Source: CAD feature listing. Evaluate the final solid. Frame: model axes, mm. Face numbers are marked on the shaded views. Round coordinates to 2 decimals unless told otherwise and drop trailing zeros. Write each loop counter-clockwise with the first axis right and the second up, starting at its lowest first coordinate (ties: lowest second). Pieces come first, ordered by that corner, then holes. Notation, with made-up numbers: M 85,-18.75 L 139,-18.75 A14 ccw 139,7.25 Z; hole C 73.25,41.5 d8. An arc over 180 degrees is marked long. Use a Markdown table: item, result.
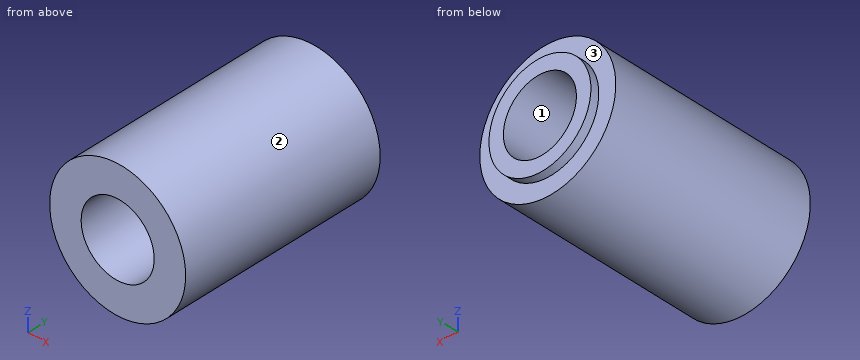
```python
from build123d import *

# Parameters (mm, degrees)
SKETCH1_R            = 4
BOSS_EXTRUDE1_DEPTH  = 12.82
SKETCH2_OUTSIDE_W    = 13.42
SKETCH2_OUTSIDE_H    = 13.42
SKETCH2_OUTSIDE_R    = 3
CUT_EXTRUDE1_DEPTH   = 0.5
M4_CLEARANCE_HOLE1_D = 4.3


with BuildPart() as part:
    # Sketch1 → Boss-Extrude1 (new body)
    with BuildSketch(Plane(origin=(0, 0, 0), x_dir=(1, 0, 0), z_dir=(0, 1, 0))):
        Circle(SKETCH1_R)
    extrude(amount=BOSS_EXTRUDE1_DEPTH)

    # Sketch2 outside → Cut-Extrude1 (cut)
    with BuildSketch(Plane(origin=(0, 12.82, 0), x_dir=(1, 0, 0), z_dir=(0, 1, 0))):
        Rectangle(SKETCH2_OUTSIDE_W, SKETCH2_OUTSIDE_H)
        Circle(SKETCH2_OUTSIDE_R, mode=Mode.SUBTRACT)
    extrude(amount=-CUT_EXTRUDE1_DEPTH, mode=Mode.SUBTRACT)

    # M4 Clearance Hole1 (through all)
    with Locations(Plane(origin=(0, 12.82, 0), x_dir=(1, 0, 0), z_dir=(0, 1, 0))):
        with Locations((0, 0)):
            Hole(M4_CLEARANCE_HOLE1_D / 2)


solid = part.part
```
Q1. Mould query, pull axis X, two halves, no side actions, for the marked faces 1, 2 and 3. Classes: +X half, -X half, draft (parallel to the pull), parting line (faces both ways), or undercut.
Results are:
| item | result |
|---|---|
| face 1 | undercut |
| face 2 | parting line |
| face 3 | draft |
Q2. Section D-D on x = -2.75. Return loops of the section in (y, z).
Results are:
| item | result |
|---|---|
| outline | M 0,-2.9 L 12.32,-2.9 L 12.32,-1.2 L 12.82,-1.2 L 12.82,1.2 L 12.32,1.2 L 12.32,2.9 L 0,2.9 Z |
Q3. Section C-C on y = 4. Return loops of the section in (x, z), plus the area to 3 significant figures.
Results are:
| item | result |
|---|---|
| outline | C 0,0 d8; hole C 0,0 d4.3 |
| area | 35.7 mm^2 |
Q4. First-contact query: pin 1 Ø3 at (y, z) = (9.5, -2) entering from -X. Flat tip, straight axial feed; report the tip coordinate or a pass-through.
Results are:
| item | result |
|---|---|
| pin 1 | x = -3.97 |
Q5. Line query: L1, parallel to Z at x = 0, y = 9.5; L2, parallel to Z at x = -0.75, y = 7.75; L3, parallel to X at y = 8, z = -1.25. Output: solid intervals per line, ascending.
Results are:
| item | result |
|---|---|
| L1 | -4 to -2.15, 2.15 to 4 |
| L2 | -3.93 to -2.01, 2.01 to 3.93 |
| L3 | -3.8 to -1.75, 1.75 to 3.8 |
Q6. Section A-A on z = 0. Return loops of the section in (x, y), plus the area to 3 significant figures.
Results are:
| item | result |
|---|---|
| outline | M -4,0 L -2.15,0 L -2.15,12.82 L -3,12.82 L -3,12.32 L -4,12.32 Z; M 2.15,0 L 4,0 L 4,12.32 L 3,12.32 L 3,12.82 L 2.15,12.82 Z |
| area | 46.4 mm^2 |
Q7. Section B-B on x = 0. Return loops of the section in (y, z), plus the area to 3 significant figures.
Results are:
| item | result |
|---|---|
| outline | M 0,-4 L 12.32,-4 L 12.32,-3 L 12.82,-3 L 12.82,-2.15 L 0,-2.15 Z; M 0,2.15 L 12.82,2.15 L 12.82,3 L 12.32,3 L 12.32,4 L 0,4 Z |
| area | 46.4 mm^2 |
